Geometry check sheet. Reference: the model listing, model coordinates, mm. Face numbers are marked on the shaded views. A direction names the side the tool comes from. Round coordinates to 2 decimals unless told otherwise and drop trailing zeros. Loops run counter-clockwise (first coordinate to the right, second up) from the corner with the lowest first, then second, coordinate; pieces in that order, holes last. Notation, with made-up numbers: M 38,-33 L 72,-33 A24 cw 72,-21 Z; hole C -15.5,6 d9. An arc over 180 degrees is marked long. Use one line per item in the form item = value. Start each with the question number.
1. Cross-section at D-D (y = 67). Record the boundary of the cut face in (x, z).
2. Draft check along X on the marked faces 5, 6, 7 and 8. Enter one of: pulls with the +X half, pulls with the -X half, needs draft (parallel to the pull), parting line crosses it, or undercut.
3. Go/stop test with flat-tipped pins: pin 1 (4 mm diameter, centred on x = -39.22, y = 59.22, fed in from +Z); pin 2 (7 mm diameter, centred on x = -51.5, y = 50, fed in from -Z). Record where each tip stops, or that it passes through.
4. Cross-section at B-B (y = 56.5). Record the boundary of the cut face in (x, z).
5. Material ranges on line 1 (Z direction, x = -38, y = 75); line 2 (Z direction, x = -47.5, y = 52); line 3 (X direction, y = 56, z = 4.75), recorded low to high.
6. Set-up check for the marked faces 1, 2, 3 and 4: record each of +Z, -Z, +X, -X, +Y, -Y from which the full face is reachable in a straight line by a thin tool's end or side.
7. Cross-section at C-C (z = 5). Record the boundary of the cut face in (x, y) (1 decimal), then the cut area to 3 significant figures.
8. Cross-section at A-A (x = -50). Record the boundary of the cut face in (y, z), then the cut area to 3 significant figures.
```python
from build123d import *

# Parameters (mm, degrees)
F0_W     = 28.448
F0_H     = 44.8691
F0_R     = 1.5875
F0_R_2   = 2.54
F1_DEPTH = 6.35
F3_DEPTH = 38.1
F5_DEPTH = 50.8
F6_R     = 1.905
F7_DEPTH = 2.54


with BuildPart() as f1:
    # F0 (on Top) → F1 (new body)
    with BuildSketch(Plane.XY):
        with Locations((-49.5780322009, 62.1553933926)):
            Rectangle(F0_W, F0_H)
        with Locations((-60.3500753641, 59.2026433926)):
            Circle(F0_R, mode=Mode.SUBTRACT)
        with Locations((-50.499536097, 58.2501433926)):
            Circle(F0_R_2, mode=Mode.SUBTRACT)
        with Locations((-39.2191149294, 59.2153433926)):
            Circle(F0_R, mode=Mode.SUBTRACT)
    extrude(amount=F1_DEPTH)

    # F2 (on face) → F3 (join)
    with BuildSketch(Plane.XZ.offset(-39.7208433926)):
        Polygon((-56.1168316064, 0), (-60.7346379378, 0), (-60.7346379378, -2.54), (-58.9566379378, -2.54), align=None)
        Polygon((-40.6839104433, 0), (-45.3017167747, 0), (-42.4619104433, -2.54), (-40.6839104433, -2.54), align=None)
    extrude(amount=-F3_DEPTH)

    # F4 (on face) → F5 (cut)
    with BuildSketch(Plane.YZ.offset(-35.3540322009)):
        Polygon((63.5858905178, -2.54), (77.8208433926, -2.54), (77.8208433926, 1.5875), (61.6612056587, 1.5875), align=None)
        Polygon((39.7208433926, 0), (39.7208433926, -2.54), (52.1558905178, -2.54), (53.3403119695, 0), align=None)
    extrude(amount=-F5_DEPTH, mode=Mode.SUBTRACT)

    # F6 (on face) + F3_face (on face) → F7 (join)
    with BuildSketch(Plane.XY.offset(6.35)):
        with Locations((-61.2620322009, 81.3514433926)):
            Circle(F6_R)
        with Locations((-37.8940322009, 81.3514433926)):
            Circle(F6_R)
    with BuildSketch(Plane(origin=(-59.8787005815, 59.2026433926, 0), x_dir=(1, 0, 0), z_dir=(0, 0, 1))):
        with BuildLine():
            Line((-0.8559373563, 1.5402168279), (-0.8559373563, -1.5402168279))
            ThreePointArc((-0.8559373563, -1.5402168279), (0.5057800578, -1.251129357), (1.1161252174, 0))
            ThreePointArc((1.1161252174, 0), (0.5057800578, 1.251129357), (-0.8559373563, 1.5402168279))
        make_face()
    extrude(amount=F7_DEPTH)


solid = f1.part
```
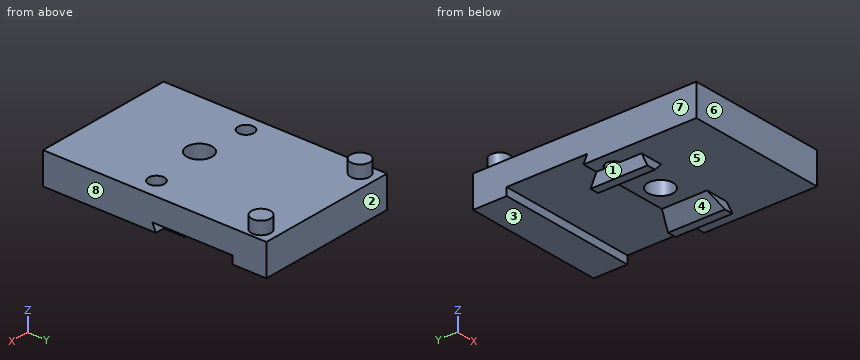
Reported:
q1.outline = M -63.8,1.59 L -35.35,1.59 L -35.35,6.35 L -63.8,6.35 Z
q2.face_5 = undercut
q2.face_6 = needs draft
q2.face_7 = pulls with the -X half
q2.face_8 = pulls with the +X half
q3.pin_1 = 6.35
q3.pin_2 = 0
q4.outline = M -63.8,0 L -60.73,0 L -60.73,-2.54 L -58.96,-2.54 L -56.12,0 L -52.34,0 L -52.34,6.35 L -63.8,6.35 Z; M -48.66,0 L -45.3,0 L -42.46,-2.54 L -40.68,-2.54 L -40.68,0 L -35.35,0 L -35.35,6.35 L -48.66,6.35 Z
q5.line_1 = 1.59 to 6.35
q5.line_2 = 0 to 6.35
q5.line_3 = -63.8 to -51.68, -49.32 to -35.35
q6.face_1 = -Z
q6.face_2 = +Z, -Z, +X, -X, +Y
q6.face_3 = -Z, +X, -X, +Y
q6.face_4 = -Z, +Y, -Y
q7.outline = M -63.8,39.7 L -35.4,39.7 L -35.4,84.6 L -63.8,84.6 Z; hole C -60.4,59.2 d3.2; hole C -50.5,58.3 d5.1; hole C -39.2,59.2 d3.2
q7.area = 1,240 mm²
q8.outline = M 39.72,0 L 55.76,0 L 55.76,6.35 L 39.72,6.35 Z; M 60.74,0 L 62.4,0 L 61.66,1.59 L 77.82,1.59 L 77.82,0 L 84.59,0 L 84.59,6.35 L 60.74,6.35 Z
q8.area = 228 mm²
